Geometry check sheet. Reference: the model listing, model coordinates, mm. A direction names the side the tool comes from. Coordinates: 2 decimals unless noted, no trailing zeros. Write each loop counter-clockwise with the first axis right and the second up, starting at its lowest first coordinate (ties: lowest second). Pieces come first, ordered by that corner, then holes. Notation, with made-up numbers: (71, 0.25) -> (110, 0.25) arc R23 cw to (110, 27.25) -> close; hole circle Ø11 at (-30, -23). An arc over 180 degrees is marked (long way). Use a Markdown table: item, result.
Autodesk Inventor part; units mm, degrees
ref_plane "YZ Plane" through (0, 0, 0) normal (1, 0, 0) x (0, 1, 0)
ref_plane "XZ Plane" through (0, 0, 0) normal (0, 1, 0) x (-1, 0, 0)
ref_plane "XY Plane" through (0, 0, 0) normal (0, 0, 1) x (1, 0, 0)
sketch "Sketch1" plane through (0, 0, 0) normal (0, 0, 1) x (1, 0, 0)
  line L0 (1.5, 2) -> (-1.5, 2) construction
  arc A0 (-1.5, 2) -> (1.5, 2) centre (0, 0) ccw construction
  circle A1 centre (0, 0) radius 11 construction
  arc A2 (-1.5, 2) -> (1.5, 2) centre (0, 0) ccw construction
  line L1 (1.5, 2) -> (-1.5, 2) construction
  circle A3 centre (0, 0) radius 4.6
  arc A4 (-1.533, 2.1) -> (1.533, 2.1) centre (0, 0) ccw
  line L2 (-1.533, 2.1) -> (1.533, 2.1)
  dimension "d0" = 9.2
  dimension "d1" = 5.2
  dimension "d2" = 0.1
extrude "Extrusion1" add sketch "Sketch1" along normal blind 12
sketch "Sketch2" plane through (0, 0, 0) normal (1, 0, 0) x (0, 1, 0)
  line L0 (0, 12.2) -> (21, 12.2) construction
  line L1 (8.4705, 1) -> (21, 1) construction
  line L2 (0, -2.44) -> (0, 14.64)
  line L3 (4.6, 0) -> (4.6, 12) construction
  line L4 (4.6, 10.36) -> (3.8845, 10.36) construction
  line L5 (4.6, 0) -> (4.6, 12) construction
  line L6 (4.6, 9.56) -> (3.8621, 9.56) construction
  line L7 (4.6, 10.36) -> (4, 10.04)
  line L8 (4, 10.04) -> (4, 9.88)
  line L9 (4.6, 0) -> (4.6, 12) construction
  line L10 (4, 9.88) -> (4.6, 9.56)
  line L11 (4.6, 9.56) -> (4.6, 9.4)
  line L12 (4.6, 0) -> (4.6, 12) construction
  line L13 (4.6, 9.4) -> (4, 9.08)
  line L14 (4, 9.08) -> (4, 8.92)
  line L15 (4, 8.92) -> (4.6, 8.6)
  line L16 (4.6, 8.6) -> (4.6, 8.44)
  line L17 (4.6, 8.44) -> (4, 8.12)
  line L18 (4, 8.12) -> (4, 7.96)
  line L19 (4, 7.96) -> (4.6, 7.64)
  line L20 (4.6, 7.64) -> (4.6, 7.48)
  line L21 (4.6, 7.48) -> (4, 7.16)
  line L22 (4, 7.16) -> (4, 7)
  line L23 (4, 7) -> (4.6, 6.68)
  line L24 (4.6, 6.68) -> (4.6, 6.52)
  line L25 (4.6, 6.52) -> (4, 6.2)
  line L26 (4, 6.2) -> (4, 6.04)
  line L27 (4, 6.04) -> (4.6, 5.72)
  line L28 (4.6, 5.72) -> (4.6, 5.56)
  line L29 (4.6, 5.56) -> (4, 5.24)
  line L30 (4, 5.24) -> (4, 5.08)
  line L31 (4, 5.08) -> (4.6, 4.76)
  line L32 (4.6, 4.76) -> (4.6, 4.6)
  line L33 (4.6, 4.6) -> (4, 4.28)
  line L34 (4, 4.28) -> (4, 4.12)
  line L35 (4, 4.12) -> (4.6, 3.8)
  line L36 (4.6, 3.8) -> (4.6, 3.64)
  line L37 (4.6, 3.64) -> (4, 3.32)
  line L38 (4, 3.32) -> (4, 3.16)
  line L39 (4, 3.16) -> (4.6, 2.84)
  line L40 (4.6, 2.84) -> (4.6, 2.68)
  line L41 (4.6, 10.36) -> (4.6, 12.2) construction
  line L42 (4.6, 10.36) -> (6.2592, 10.36) construction
  line L43 (6.2592, 10.36) -> (6.2592, 12.2) construction
  line L44 (4.6, 2.84) -> (5.8943, 2.84) construction
  line L45 (5.8943, 2.84) -> (5.8943, 1) construction
  line L46 (4.6, 10.36) -> (4.6, 9.56)
  line L47 (4.6, 9.4) -> (4.6, 8.6)
  line L48 (4.6, 8.44) -> (4.6, 7.64)
  line L49 (4.6, 7.48) -> (4.6, 6.68)
  line L50 (4.6, 0) -> (4.6, 12)
  line L51 (4.6, 6.52) -> (4.6, 5.72)
  line L52 (4.6, 0) -> (4.6, 12)
  line L53 (4.6, 5.56) -> (4.6, 4.76)
  line L54 (4.6, 4.6) -> (4.6, 3.8)
  line L55 (4.6, 0) -> (4.6, 12)
  line L56 (4.6, 3.64) -> (4.6, 2.84)
  line L57 (4.6, 0) -> (4.6, 12)
  point P0 (0, 0)
  dimension "d6" = 0.8
  dimension "d7" = 0.16
  dimension "d8" = 0.6
  dimension "d9" = 0.16
  dimension "d12" = 0.96
revolve "Revolution1" cut sketch "Sketch2" angle 360 about axis through (0, 0, -10) along (0, 0, 1)
sketch "Sketch3" plane through (0, 0, 0) normal (0, 0, -1) x (-1, 0, 0)
  circle A0 centre (0, 0) radius 4.6
  circle A1 centre (0, 0) radius 6.6
  dimension "d17" = 2
extrude "Extrusion2" add sketch "Sketch3" against normal blind 1
properties part number "NewDriveWheel2"
Item 1: Section check C-C on x = 5.25. Record the boundary of the cut face in (y, z).
Answer block:
| item | result |
|---|---|
| outline | (-4, 0) -> (4, 0) -> (4, 1) -> (-4, 1) -> close |
Item 2: Section check A-A on z = 2. Record the boundary of the cut face in (x, y).
Answer block:
| item | result |
|---|---|
| outline | circle Ø9.2 at (0, 0); hole (-1.53, 2.1) arc R2.6 ccw (long way) to (1.53, 2.1) -> close |
Item 3: Depth check by flat-ended pin: P1, Ø6, axis at x = 0, z = 8.5, coming from the -Y side; P2, Ø1.5, axis at x = 1.5, z = 5.5, coming from the +Y side; P3, Ø2, axis at y = 5, z = 3.5, coming from the +X side. Enter the tip coordinate at first touch or a pass-through.
Answer block:
| item | result |
|---|---|
| P1 | stops at y = -4.6 |
| P2 | stops at y = 4.54 |
| P3 | stops at x = 2.25 |
Item 4: Section check B-B on y = 5.5. Record the boundary of the cut face in (x, z), then the cut area to 3 significant figures.
Answer block:
| item | result |
|---|---|
| outline | (-3.65, 0) -> (3.65, 0) -> (3.65, 1) -> (-3.65, 1) -> close |
| area | 7.30 mm^2 |
Item 5: Thickness scan on L1, parallel to X at y = 0, z = 8.5; L2, parallel to Y at x = 0, z = 8; L3, parallel to Z at x = 4.25, y = -4.25. Record the ranges inside material, lowest first. Write a range as [from, to].
Answer block:
| item | result |
|---|---|
| L1 | x = [-4.6, -2.6], [2.6, 4.6] |
| L2 | y = [-4, -2.6], [2.1, 4] |
| L3 | z = [0, 1] |
Item 6: Tool access check on faces 1 (the flat face through (-3, 0, 0)), 2 (the cylindrical face through (-3.65, 2.8, 11.17)). Record the directions out of +Z, -Z, +X, -X, +Y, -Y that give a thin tool (end or side, any length) a straight path to the whole face; none if there is none.
Answer block:
| item | result |
|---|---|
| face 1 | -Z, +X, -X, +Y, -Y |
| face 2 | +Z |
